CAD build for the part. Positions are in the model's coordinates, mm. A direction names the side the tool comes from. Coordinates: 2 decimals unless noted, no trailing zeros. Order: outer loops, then holes, each group sorted by start corner. A loop starts at its lowest first (then second) coordinate and runs counter-clockwise, first axis right, second up. Notation, with made-up numbers: (36.25, 60.5) - (90.25, 60.5) arc R37 ccw to (90.25, 96.5) - close; hole circle Ø2 at (84, 29.5). An arc over 180 degrees is marked (long way). Write each question's results on one line, items separated by ' | '. Start each with the question number.
Q1. Which spindle directions (+Z, -Z, +X, -X, +Y, -Y) get a long thin tool onto all of the face, cutting with end or side? Do faces 1 (the flat face through (74.603, -5, -47)), 2 (the flat face through (28.7, 7, 42)), 3 (the cylindrical face through (7.167, -13.496, 4.677)), 4 (the flat face through (-6, -15, 5)). Say none if no direction does.
Q2. Band-saw the part on B-B, the plane x = 37. Write the cut outline in (y, z), then the cut area to 3 significant figures.
Q3. Wall check: probe 1 along Z at (x, y) = (63, 3); probe 2 along X at (y, z) = (-0.5, 42); probe 3 along X at (y, z) = (2.75, -40). Give the ranges that are in metal, low to high.
Q4. Band-saw the part on A-A, the plane z = 40. Count the separate pieces of the cut face and the enclosed holes in it, then the cut area to 3 significant figures.
Q5. Band-saw the part on C-C, the plane z = 27. Write the cut outline in (x, y), then the cut area to 3 significant figures.
Q6. Pin check, flat tips, straight feed: P1, Ø1.5, axis at x = 19.5, y = -5.5, coming from the -Z side; P2, Ø1.5, axis at y = -7, z = 4, coming from the -X side; P3, Ø7, axis at x = 62.6, z = 40, coming from the -Y side; P4, Ø6.5, axis at y = -11, z = -45, coming from the -X side. Stop position of each tip, or through.
Q7. Pull direction X, two halves, no side cores. Call faces 5 (the flat face through (-33.155, 4.93, 43.379)), 6 (the flat face through (-48.527, 8.028, -20.67)), 7 (the flat face through (95.08, -7.6, -43.79)): released by +X, released by -X, zero draft, split by the parting line, or undercut.
```python
from build123d import *

# Parameters (mm, degrees)
SKETCH1_R            = 5.05
SKETCH1_R_2          = 6
SKETCH1_R_3          = 2.6
BOSS_EXTRUDE1_DEPTH  = 10
SKETCH3_W            = 25
SKETCH3_H            = 5
BOSS_EXTRUDE3_DEPTH  = 20
FILLET2_R            = 5
SKETCH4_R            = 2.75
CUT_EXTRUDE1_DEPTH   = 20
RIB9_REACH           = 120.579
SKETCH10_WALL_W      = 258.738758418
SKETCH10_WALL_H      = 3
RIB10_START          = -3
RIB10_DEPTH          = 3
SKETCH12_W           = 25
SKETCH12_H           = 5
BOSS_EXTRUDE4_DEPTH  = 20
FILLET3_R            = 5
SKETCH13_R           = 2.75
CUT_EXTRUDE2_DEPTH   = 145.073688744
RIB11_REACH          = 188.093
SKETCH14_WALL_W      = 393.76792997
SKETCH14_WALL_H      = 3
RIB12_REACH          = 164.552
SKETCH15_WALL_W      = 347.125659706
SKETCH15_WALL_H      = 3
FILLET2_OF_MIRROR3_R = 5
FILLET3_OF_MIRROR3_R = 5
SKETCH16_W           = 29.246937375
SKETCH16_H           = 5
BOSS_EXTRUDE5_DEPTH  = 15
FILLET4_R            = 5
CUT_EXTRUDE3_REACH   = 116.006
SKETCH17_R           = 1.25
CUT_EXTRUDE4_DEPTH   = 4
CUT_EXTRUDE5_DEPTH   = 3


# Read off the part's stored shape, not the designer's step: Rib10
with BuildPart() as part:
    # Sketch1 → Boss-Extrude1 (new body)
    with BuildSketch(Plane(origin=(0, 0, 0), x_dir=(1, 0, 0), z_dir=(0, 1, 0))):
        with BuildLine():
            Line((-6.527225889, 55), (-59.0480575, 32.078029865))
            ThreePointArc((-59.0480575, 32.078029865), (-80.0480575, 0), (-59.0480575, -32.078029865))
            Line((-59.0480575, -32.078029865), (-6.527225889, -55))
            Line((-6.527225889, -55), (96.603456399, -55))
            Line((96.603456399, -55), (96.603456399, -40))
            Line((96.603456399, -40), (96.603456399, 55))
            Line((96.603456399, 55), (-6.527225889, 55))
        make_face()
        with Locations(Location((46.603456399, 40, 0), (0, 0, 270))):
            Circle(SKETCH1_R, mode=Mode.SUBTRACT)
        with Locations(Location((46.603456399, -40, 0), (0, 0, 270))):
            Circle(SKETCH1_R, mode=Mode.SUBTRACT)
        with Locations(Location((-45.0480575, 0, 0), (0, 0, 270))):
            Circle(SKETCH1_R_2, mode=Mode.SUBTRACT)
        with Locations(Location((30.603456399, 40, 0), (0, 0, 270))):
            Circle(SKETCH1_R_3, mode=Mode.SUBTRACT)
        with Locations(Location((62.603456399, 40, 0), (0, 0, 270))):
            Circle(SKETCH1_R_3, mode=Mode.SUBTRACT)
        with Locations(Location((30.603456399, -40, 0), (0, 0, 270))):
            Circle(SKETCH1_R_3, mode=Mode.SUBTRACT)
        with Locations(Location((62.603456399, -40, 0), (0, 0, 270))):
            Circle(SKETCH1_R_3, mode=Mode.SUBTRACT)
        with Locations(Location((-45.0480575, 18.5, 0), (0, 0, 270))):
            Circle(SKETCH1_R_3, mode=Mode.SUBTRACT)
        with Locations(Location((-45.0480575, -18.5, 0), (0, 0, 270))):
            Circle(SKETCH1_R_3, mode=Mode.SUBTRACT)
    extrude(amount=BOSS_EXTRUDE1_DEPTH)

    # Sketch3 → Boss-Extrude3 (add)
    with BuildSketch(Plane.XZ):
        with Locations((5.972774111, -52.5)):
            Rectangle(SKETCH3_W, SKETCH3_H)
    boss_extrude3 = extrude(amount=BOSS_EXTRUDE3_DEPTH)

    # Fillet2
    fillet2_edges = [part.edges().sort_by_distance(p)[0] for p in [
        (-6.527225889, -20, -52.5),
        (18.472774111, -20, -52.5),
    ]]
    fillet(fillet2_edges, radius=FILLET2_R)

    # Sketch4 → Cut-Extrude1 (cut)
    with BuildSketch(Plane.XY.offset(-50)):
        with Locations((5.972774111, -12)):
            Circle(SKETCH4_R)
    cut_extrude1 = extrude(amount=-CUT_EXTRUDE1_DEPTH, mode=Mode.SUBTRACT)

    # Sketch10 wall → Rib9 (add, up to next)
    with BuildSketch(Plane(origin=(-6.527225889, -7.5, -43.706752766), x_dir=(0, 0.76604444311, 0.642787609697), z_dir=(0, 0.642787609697, -0.76604444311)), mode=Mode.PRIVATE) as rib9_sk1:
        with Locations((0, 1.5)):
            Rectangle(SKETCH10_WALL_W, SKETCH10_WALL_H)
    rib9_tool1 = extrude(rib9_sk1.sketch, amount=RIB9_REACH, mode=Mode.PRIVATE) - part.part
    rib9 = rib9_tool1.solids().sort_by_distance((-6.527225889, -7.5, -43.706752766))[0]
    add(rib9)

    # Rib10 outline → Rib10 (add)
    with BuildSketch(Plane(origin=(18.472774111, 0, 0), x_dir=(0, 0, -1), z_dir=(1, 0, 0)).offset(RIB10_START)):
        Polygon((37.413505532, 0), (50, -15), (50, 0), align=None)
    rib10 = extrude(amount=RIB10_DEPTH)

    # Sketch12 → Boss-Extrude4 (add)
    with BuildSketch(Plane.XZ):
        with Locations((84.103456399, -52.5)):
            Rectangle(SKETCH12_W, SKETCH12_H)
    boss_extrude4 = extrude(amount=BOSS_EXTRUDE4_DEPTH)

    # Fillet3
    fillet3_edges = [part.edges().sort_by_distance(p)[0] for p in [
        (96.603456399, -20, -52.5),
        (71.603456399, -20, -52.5),
    ]]
    fillet(fillet3_edges, radius=FILLET3_R)

    # Sketch13 → Cut-Extrude2 (cut, through all)
    with BuildSketch(Plane.XY.offset(-50)):
        with Locations((84.103456399, -12)):
            Circle(SKETCH13_R)
    cut_extrude2 = extrude(amount=-CUT_EXTRUDE2_DEPTH, mode=Mode.SUBTRACT)

    # Sketch14 wall → Rib11 (add, up to next)
    with BuildSketch(Plane(origin=(96.603456399, -7.5, -43.706752766), x_dir=(0, 0.76604444311, 0.642787609697), z_dir=(0, -0.642787609697, 0.76604444311)), mode=Mode.PRIVATE) as rib11_sk1:
        with Locations((0, 1.5)):
            Rectangle(SKETCH14_WALL_W, SKETCH14_WALL_H)
    rib11_tool1 = extrude(rib11_sk1.sketch, amount=-RIB11_REACH, mode=Mode.PRIVATE) - part.part
    rib11 = rib11_tool1.solids().sort_by_distance((96.603456399, -7.5, -43.706752766))[0]
    add(rib11)

    # Sketch15 wall → Rib12 (add, up to next)
    with BuildSketch(Plane(origin=(71.603456399, -7.331327668, -43.565219875), x_dir=(0, 0.766044443114, 0.642787609692), z_dir=(0, 0.642787609692, -0.766044443114)), mode=Mode.PRIVATE) as rib12_sk1:
        with Locations((0, 1.5)):
            Rectangle(SKETCH15_WALL_W, SKETCH15_WALL_H)
    rib12_tool1 = extrude(rib12_sk1.sketch, amount=RIB12_REACH, mode=Mode.PRIVATE) - part.part
    rib12 = rib12_tool1.solids().sort_by_distance((71.603456399, -7.331327668, -43.565219875))[0]
    add(rib12)

    # Mirror3: Boss-Extrude3, Cut-Extrude1, Rib9, Rib10, Boss-Extrude4, Cut-Extrude2, Rib11, Rib12 across plane
    add(boss_extrude3.mirror(Plane.XY))
    add(cut_extrude1.mirror(Plane.XY), mode=Mode.SUBTRACT)
    add(rib9.mirror(Plane.XY))
    add(rib10.mirror(Plane.XY))
    add(boss_extrude4.mirror(Plane.XY))
    add(cut_extrude2.mirror(Plane.XY), mode=Mode.SUBTRACT)
    add(rib11.mirror(Plane.XY))
    add(rib12.mirror(Plane.XY))

    # Fillet2 of Mirror3
    fillet2_of_mirror3_edges = [part.edges().sort_by_distance(p)[0] for p in [
        (-6.527225889, -20, 52.5),
        (18.472774111, -20, 52.5),
    ]]
    fillet(fillet2_of_mirror3_edges, radius=FILLET2_OF_MIRROR3_R)

    # Fillet3 of Mirror3
    fillet3_of_mirror3_edges = [part.edges().sort_by_distance(p)[0] for p in [
        (96.603456399, -20, 52.5),
        (71.603456399, -20, 52.5),
    ]]
    fillet(fillet3_of_mirror3_edges, radius=FILLET3_OF_MIRROR3_R)

    # Sketch16 → Boss-Extrude5 (add)
    with BuildSketch(Plane.XZ):
        with Locations((-6.030626379, 4.641549892)):
            Rectangle(SKETCH16_W, SKETCH16_H)
    extrude(amount=BOSS_EXTRUDE5_DEPTH)

    # Fillet4
    fillet4_edges = [part.edges().sort_by_distance(p)[0] for p in [
        (8.592842309, -15, 4.641549892),
        (-20.654095066, -15, 4.641549892),
    ]]
    fillet(fillet4_edges, radius=FILLET4_R)

    # Sketch17 → Cut-Extrude3 (cut, up to next)
    with BuildSketch(Plane(origin=(0, 0, 2.141549892), x_dir=(-1, 0, 0), z_dir=(0, 0, -1)), mode=Mode.PRIVATE) as cut_extrude3_sk1:
        with Locations((0, -10.207909403)):
            Circle(SKETCH17_R)
    cut_extrude3_tool1 = extrude(cut_extrude3_sk1.sketch, amount=-CUT_EXTRUDE3_REACH, mode=Mode.PRIVATE) & part.part
    # Sketch17 → Cut-Extrude3 (cut, up to next)
    with BuildSketch(Plane(origin=(0, 0, 2.141549892), x_dir=(-1, 0, 0), z_dir=(0, 0, -1)), mode=Mode.PRIVATE) as cut_extrude3_sk2:
        with Locations((9.5, -10.207909403)):
            Circle(SKETCH17_R)
    cut_extrude3_tool2 = extrude(cut_extrude3_sk2.sketch, amount=-CUT_EXTRUDE3_REACH, mode=Mode.PRIVATE) & part.part
    add(cut_extrude3_tool1.solids().sort_by_distance((0, -10.207909, 2.14155))[0], mode=Mode.SUBTRACT)
    add(cut_extrude3_tool2.solids().sort_by_distance((-9.5, -10.207909, 2.14155))[0], mode=Mode.SUBTRACT)

    # Sketch19 → Cut-Extrude4 (cut)
    with BuildSketch(Plane(origin=(0, 10, 0), x_dir=(1, 0, 0), z_dir=(0, 1, 0))):
        Polygon((-42.788929966, 14.33951011), (-40.315403797, 18.37621689), (-42.57453133, 22.536706779), (-47.307185033, 22.66048989), (-49.780711203, 18.62378311), (-47.52158367, 14.463293221), align=None)
        Polygon((-42.729558415, -22.627698551), (-40.314116153, -18.555970169), (-42.632615238, -14.428271618), (-47.366556585, -14.372301449), (-49.781998846, -18.444029831), (-47.463499761, -22.571728382), align=None)
    extrude(amount=-CUT_EXTRUDE4_DEPTH, mode=Mode.SUBTRACT)

    # Sketch20 → Cut-Extrude5 (cut)
    with BuildSketch(Plane(origin=(0, 10, 0), x_dir=(1, 0, 0), z_dir=(0, 1, 0))):
        Polygon((58.549967326, 37.554072841), (62.694946918, 35.266611909), (66.748435991, 37.712539068), (66.656945472, 42.445927159), (62.51196588, 44.733388091), (58.458476807, 42.287460932), align=None)
        Polygon((26.494447933, 37.648536039), (30.585379692, 35.265762304), (34.694388158, 37.617226264), (34.712464865, 42.351463961), (30.621533106, 44.734237696), (26.51252464, 42.382773736), align=None)
        Polygon((58.549967326, -37.554072841), (58.458476807, -42.287460932), (62.51196588, -44.733388091), (66.656945472, -42.445927159), (66.748435991, -37.712539068), (62.694946918, -35.266611909), align=None)
        Polygon((26.494447933, -37.648536039), (26.51252464, -42.382773736), (30.621533106, -44.734237696), (34.712464865, -42.351463961), (34.694388158, -37.617226264), (30.585379692, -35.265762304), align=None)
    extrude(amount=-CUT_EXTRUDE5_DEPTH, mode=Mode.SUBTRACT)


solid = part.part
```
Results below:
1) face 1: -Y | face 2: +Y | face 3: +X, -Y | face 4: +X, -X, -Y
2) outline: (0, -55) - (10, -55) - (10, 55) - (0, 55) - close | area: 1,100 mm²
3) probe 1: z = -55 to -42.57, -37.43 to 37.43, 42.57 to 55 | probe 2: x = -6.53 to -3.53, 15.47 to 18.47, 71.6 to 74.6, 93.6 to 96.6 | probe 3: x = -40.9 to 28, 33.2 to 41.55, 51.65 to 60, 65.2 to 96.6
4) separate pieces: 4 | enclosed holes: 0 | area: 1,190 mm²
5) outline: (-67.32, 0) - (96.6, 0) - (96.6, 10) - (-67.32, 10) - close | area: 1,640 mm²
6) P1: passes through | P2: stops at x = -20.65 | P3: stops at y = 0 | P4: stops at x = -6.53
7) face 5: released by -X | face 6: undercut | face 7: zero draft
